from build123d import *

# Parameters (mm, degrees)
SKETCH1_W                      = 60
SKETCH1_H                      = 77
BOSS_EXTRUDE1_DEPTH            = 10
SKETCH2_W                      = 60
SKETCH2_H                      = 12
BOSS_EXTRUDE2_DEPTH            = 52
SKETCH3_W                      = 60
SKETCH3_H                      = 33
BOSS_EXTRUDE3_DEPTH            = 15
M5X0_8_TAPPED_HOLE1_D          = 4.2
CBORE_FOR_M5_SHCS1_D           = 5.5
CBORE_FOR_M5_SHCS1_CBORE_D     = 10
CBORE_FOR_M5_SHCS1_CBORE_DEPTH = 20
CBORE_FOR_M3_SHCS1_D           = 3.4
CBORE_FOR_M3_SHCS1_CBORE_D     = 6.5
CBORE_FOR_M3_SHCS1_CBORE_DEPTH = 3


with BuildPart() as part:
    # Sketch1 → Boss-Extrude1 (new body)
    with BuildSketch(Plane(origin=(0, 0, 0), x_dir=(1, 0, 0), z_dir=(0, 1, 0))):
        with Locations((30, 38.5)):
            Rectangle(SKETCH1_W, SKETCH1_H)
    extrude(amount=BOSS_EXTRUDE1_DEPTH)

    # Sketch2 → Boss-Extrude2 (add)
    with BuildSketch(Plane(origin=(0, 10, 0), x_dir=(1, 0, 0), z_dir=(0, 1, 0))):
        with Locations((30, 71)):
            Rectangle(SKETCH2_W, SKETCH2_H)
    extrude(amount=BOSS_EXTRUDE2_DEPTH)

    # Sketch3 → Boss-Extrude3 (add)
    with BuildSketch(Plane(origin=(0, 10, 0), x_dir=(1, 0, 0), z_dir=(0, 1, 0))):
        with Locations((30, 16.5)):
            Rectangle(SKETCH3_W, SKETCH3_H)
    extrude(amount=BOSS_EXTRUDE3_DEPTH)

    # M5x0.8 Tapped Hole1 (through all)
    with Locations(Plane(origin=(0, 62, 0), x_dir=(1, 0, 0), z_dir=(0, 1, 0))):
        with Locations((18, 71), (42, 71)):
            Hole(M5X0_8_TAPPED_HOLE1_D / 2)

    # CBORE for M5 SHCS1 (through all)
    with Locations(Plane(origin=(0, 0, 0), x_dir=(-1, 0, 0), z_dir=(0, -1, 0))):
        with Locations((-42, 6), (-18, 6)):
            CounterBoreHole(CBORE_FOR_M5_SHCS1_D / 2, CBORE_FOR_M5_SHCS1_CBORE_D / 2, CBORE_FOR_M5_SHCS1_CBORE_DEPTH)

    # CBORE for M3 SHCS1 (through all)
    with Locations(Plane(origin=(0, 0, 0), x_dir=(-1, 0, 0), z_dir=(0, -1, 0))):
        with Locations((-42.5, 61.5), (-17.5, 61.5), (-17.5, 36.5), (-42.5, 36.5)):
            CounterBoreHole(CBORE_FOR_M3_SHCS1_D / 2, CBORE_FOR_M3_SHCS1_CBORE_D / 2, CBORE_FOR_M3_SHCS1_CBORE_DEPTH)


solid = part.part
Model file for the job. Use its own axes, mm. A direction names the side the tool comes from. Give positions to 0.01 mm unless a question says otherwise; leave off trailing zeros. Order: outer loops, then holes, each group sorted by start corner. A loop starts at its lowest first (then second) coordinate and runs counter-clockwise, first axis right, second up. Notation, with made-up numbers: (46, -36.75) -> (75, -36.75) arc R16 ccw to (75, -13.75) -> close; hole circle Ø5 at (85, 6). An arc over 180 degrees is marked (long way). Use CSV: the item, a comma, the result in double quotes.
1. Band-saw the part on B-B, the plane z = -71. Give the cut face in (x, y).
Outcome:
outline,"(0, 0) -> (15.9, 0) -> (15.9, 62) -> (0, 62) -> close; (20.1, 0) -> (39.9, 0) -> (39.9, 62) -> (20.1, 62) -> close; (44.1, 0) -> (60, 0) -> (60, 62) -> (44.1, 62) -> close"
2. Mould opens along X. For faces 4 (the flat face through (0, 17, -29)), 5 (the flat face through (39.8, 20, -3.8)), 6 (the flat face through (30, 12, 0)) say: +X half, -X half, draft (parallel to the pull), parting line (faces both ways), or undercut.
Outcome:
face 4,"-X half"
face 5,"undercut"
face 6,"draft"
3. Band-saw the part on D-D, the plane y = 53.5. Give the cut face in (x, z), then the cut area to 3 significant figures.
Outcome:
outline,"(0, -77) -> (60, -77) -> (60, -65) -> (0, -65) -> close; hole circle Ø4.2 at (18, -71); hole circle Ø4.2 at (42, -71)"
area,"692 mm²"
4. Drill centre lines: line 1 along X through (y, z) = (1.9, -61.5); line 2 along X through (y, z) = (48, -71); line 3 along Z through (x, y) = (18, 22). Where is each one in solid material? Low to high. Write a range as from..to.
Outcome:
line 1,"0..14.25, 20.75..39.25, 45.75..60"
line 2,"0..15.9, 20.1..39.9, 44.1..60"
line 3,"-77..-73.1, -68.9..-65, -33..-8.75, -3.25..0"
5. Band-saw the part on A-A, the plane y = 13. Give the cut face in (x, z).
Outcome:
outline,"(0, -77) -> (60, -77) -> (60, -65) -> (0, -65) -> close; (0, -33) -> (60, -33) -> (60, 0) -> (0, 0) -> close; hole circle Ø10 at (18, -6); hole circle Ø4.2 at (18, -71); hole circle Ø10 at (42, -6); hole circle Ø4.2 at (42, -71)"
6. Drop flat-ended pins along their axis: pin 1 (11.5 mm diameter, centred on x = 18, z = -6, fed in from +Y); pin 2 (8 mm diameter, centred on x = 35, y = 39, fed in from +Z); pin 3 (6 mm diameter, centred on x = 38.5, z = -12, fed in from -Y); pin 4 (4 mm diameter, centred on x = 42.5, z = -36.5, fed in from +Y). Give the stop position or say it passes through.
Outcome:
pin 1,"y = 25"
pin 2,"z = -65"
pin 3,"y = 0"
pin 4,"y = 10"
7. 3-axis set-ups, long thin cutter, end or side, ignore diameter. For faces 1 (the flat face through (30, 36, -65)), 2 (the cylindrical face through (17.923, 1.479, -64.722)), 3 (the cylindrical face through (18.3, 6.5, -35)): which of +Z, -Z, +X, -X, +Y, -Y reach the whole face in a straight line?
Outcome:
face 1,"+X, -X, +Y"
face 2,"-Y"
face 3,"+Y, -Y"
8. Band-saw the part on C-C, the plane x = 26.5. Give the cut face in (y, z), then the cut area to 3 significant figures.
Outcome:
outline,"(0, -77) -> (62, -77) -> (62, -65) -> (10, -65) -> (10, -33) -> (25, -33) -> (25, 0) -> (0, 0) -> close"
area,"1,890 mm²"
